Can you work these out from the model? Positions are in its coordinate system, mm. A direction names the side the tool comes from. Give positions to 0.01 mm unless a question says otherwise; leave off trailing zeros. Loops run counter-clockwise (first coordinate to the right, second up) from the corner with the lowest first, then second, coordinate; pieces in that order, holes last. Notation, with made-up numbers: (52.5, -5.75) - (67.5, -5.75) arc R12 cw to (67.5, -1.75) - close; hole circle Ø7 at (20, 33). An arc over 180 degrees is marked (long way). Answer as a JSON object with one key per item and string values. Group by question number.
Item 1: Suppose I cut it at D-D on z = -2.75. Write out the boundary of the cut face in (x, y).
Item 2: Will these pins go through, and if not, where does the flat tip stop? pin 1 (1.5 mm diameter, centred on y = -29.5, z = -2, fed in from -X); pin 2 (6 mm diameter, centred on y = -17.5, z = -5.5, fed in from +X); pin 3 (1 mm diameter, centred on y = -33.5, z = -0.5, fed in from +X).
Item 3: Suppose I cut it at B-B on y = 0. Write out the boundary of the cut face in (x, z).
Item 4: Suppose I cut it at A-A on x = -2.5. Write out the boundary of the cut face in (y, z).
Item 5: Which directions (+Z, -Z, +X, -X, +Y, -Y) give clear straight access to the entire face, cutting with the end or side of a thin tool? Please do faces 4 (the cylindrical face through (-4.54, -34.73, -6.03)), 5 (the flat face through (6.35, -35, 0)), 6 (the cylindrical face through (-4.44, -34.73, 6.13)), 7 (the cylindrical face through (4.54, -34.2, 6.03)).
Item 6: Thinking about a two-plate mould opening in Y: for faces 1 (the flat face through (0, -53.512, 0)), 2 (the flat face through (6, 3, 7.938)), 3 (the cylindrical face through (-1.38, -6.2, -0.11)), which applies, pulls with the +Y half, pulls with the -Y half, needs draft (parallel to the pull), parting line crosses it, or undercut?
Item 7: Please list where these lines run through material, in increasing order: L1, parallel to Y at x = 0, z = 0.25; L2, parallel to X at y = -21.5, z = -1.5; L3, parallel to Y at x = -5, z = -0.5.
from build123d import *

# Parameters (mm, degrees)
F1_R     = 6.35
F2_DEPTH = 7.9375
F3_R     = 6.34999


# Not quite as in the source:
# - a fillet or chamfer is up to 0.001 mm smaller than in the source, because OpenCascade refuses the exact size


with BuildPart() as f2:
    # F1 (on Top) → F2 (new body, symmetric)
    with BuildSketch(Plane.XY):
        with BuildLine():
            ThreePointArc((6.35, -15.4118372222), (0, 16.66875), (-6.35, -15.4118372222))
            Line((-6.35, -15.4118372222), (-6.35, -53.5118372222))
            Line((-6.35, -53.5118372222), (6.35, -53.5118372222))
            Line((6.35, -53.5118372222), (6.35, -15.4118372222))
        make_face()
        Circle(F1_R, mode=Mode.SUBTRACT)
    extrude(amount=F2_DEPTH, both=True)

    # F3 (radius 6.35 in the source; OpenCascade refuses exactly that, so slightly less here)
    f3_edges = [f2.edges().sort_by_distance(p)[0] for p in [
        (-6.35, -34.461837, -7.9375),
        (6.35, -34.461837, -7.9375),
        (-6.35, -34.461837, 7.9375),
        (6.35, -34.461837, 7.9375),
    ]]
    fillet(f3_edges, radius=F3_R)


solid = f2.part
Worked out:
{
 "1": {"outline": "(-6.24, -53.51) - (6.24, -53.51) - (6.24, -15.46) arc R16.67 ccw (long way) to (-6.24, -15.46) - close; hole circle Ø12.7 at (0, 0)"},
 "2": {"pin 1": "stops at x = -6.35", "pin 2": "stops at x = 8.22", "pin 3": "stops at x = 6.35"},
 "3": {"outline": "(-16.67, -7.94) - (-6.35, -7.94) - (-6.35, 7.94) - (-16.67, 7.94) - close; (6.35, -7.94) - (16.67, -7.94) - (16.67, 7.94) - (6.35, 7.94) - close"},
 "4": {"outline": "(-53.51, -7.42) - (-16.48, -7.42) - (-16.48, -7.94) - (-5.84, -7.94) - (-5.84, 7.94) - (-16.48, 7.94) - (-16.48, 7.42) - (-53.51, 7.42) - close; (5.84, -7.94) - (16.48, -7.94) - (16.48, 7.94) - (5.84, 7.94) - close"},
 "5": {"face 4": "-Z, -X, -Y", "face 5": "+Z, -Z, +X, -Y", "face 6": "+Z, -X, -Y", "face 7": "+Z, +X, -Y"},
 "6": {"face 1": "pulls with the -Y half", "face 2": "needs draft", "face 3": "undercut"},
 "7": {"L1": "y = -53.51 to -6.35, 6.35 to 16.67", "L2": "x = -6.35 to 6.35", "L3": "y = -53.51 to -3.91, 3.91 to 15.9"}
}
